```python
from build123d import *

# Parameters (mm, degrees)
F1_DEPTH = 15
F2_DEPTH = 2
F3_R     = 1.8
F4_DEPTH = 50


with BuildPart() as f1:
    # F0 (on Top) → F1 (new body)
    with BuildSketch(Plane.XY):
        Polygon((7.5, -12.990381), (15, 0), (7.5, 12.990381), (-7.5, 12.990381), (-15, 0), (-7.5, -12.990381), align=None)
        Polygon((6.75, 11.691343), (13.5, 0), (6.75, -11.691343), (-6.75, -11.691343), (-13.5, 0), (-6.75, 11.691343), align=None, mode=Mode.SUBTRACT)
    extrude(amount=F1_DEPTH)

    # F0 (on Top) → F2 (join)
    with BuildSketch(Plane.XY):
        Polygon((6.75, -11.691343), (13.5, 0), (6.75, 11.691343), (-6.75, 11.691343), (-13.5, 0), (-6.75, -11.691343), align=None)
    extrude(amount=F2_DEPTH)

    # F3 (on Top) → F4 (join)
    with BuildSketch(Plane.XY):
        with Locations((-11, 0)):
            Circle(F3_R)
        with Locations((5.427412, 9.569215)):
            Circle(F3_R)
        with Locations((5.408632, -9.580663)):
            Circle(F3_R)
        with Locations((0.070379, -0.000349)):
            Circle(F3_R)
    extrude(amount=-F4_DEPTH)


solid = f1.part
```
The listing builds one solid part. Answer for the finished solid, in the listing's coordinates (mm). A direction names the side the tool comes from. Give positions to 0.01 mm unless a question says otherwise; leave off trailing zeros. Order: outer loops, then holes, each group sorted by start corner. A loop starts at its lowest first (then second) coordinate and runs counter-clockwise, first axis right, second up. Notation, with made-up numbers: (-14, 53) -> (30, 53) arc R17 cw to (30, 84) -> close; hole circle Ø2 at (-9, 4). An arc over 180 degrees is marked (long way). One line per item, written item: value.
1) Find section D-D, the plane x = -11. Determine the outline of the cut face in (y, z), plus the area to 3 significant figures.
Reported:
outline: (-6.93, 0) -> (-1.8, 0) -> (-1.8, -50) -> (1.8, -50) -> (1.8, 0) -> (6.93, 0) -> (6.93, 15) -> (4.33, 15) -> (4.33, 2) -> (-4.33, 2) -> (-4.33, 15) -> (-6.93, 15) -> close
area: 275 mm^2
2) Find the intervals of material crossed by line 1 (Y direction, x = -3.5, z = 5); line 2 (X direction, y = -0.25, z = -22); line 3 (Z direction, x = -6, y = 11.5), in increasing order.
Reported:
line 1: y = -12.99 to -11.69, 11.69 to 12.99
line 2: x = -12.78 to -9.22, -1.71 to 1.85
line 3: z = 0 to 2
3) Find section C-C, the plane y = 6.25. Determine the outline of the cut face in (x, z).
Reported:
outline: (-11.39, 0) -> (11.39, 0) -> (11.39, 15) -> (9.89, 15) -> (9.89, 2) -> (-9.89, 2) -> (-9.89, 15) -> (-11.39, 15) -> close
4) Find section B-B, the plane x = -4.5. Determine the outline of the cut face in (y, z).
Reported:
outline: (-12.99, 0) -> (12.99, 0) -> (12.99, 15) -> (11.69, 15) -> (11.69, 2) -> (-11.69, 2) -> (-11.69, 15) -> (-12.99, 15) -> close
5) Find section A-A, the plane z = 7.5. Determine the outline of the cut face in (x, y), plus the area to 3 significant figures.
Reported:
outline: (-15, 0) -> (-7.5, -12.99) -> (7.5, -12.99) -> (15, 0) -> (7.5, 12.99) -> (-7.5, 12.99) -> close; hole (-13.5, 0) -> (-6.75, -11.69) -> (6.75, -11.69) -> (13.5, 0) -> (6.75, 11.69) -> (-6.75, 11.69) -> close
area: 111 mm^2
6) Flat-ended cylindrical pins translate along their axes: P1, Ø1, axis at x = 2, y = 3.5, coming from the -Z side; P2, Ø5, axis at y = 8, z = -33.5, coming from the +X side; P3, Ø5, axis at x = 6.5, z = -3, coming from the +Y side. Find the tip coordinate at first contact, or state that the pin passes through.
Reported:
P1: stops at z = 0
P2: stops at x = 7.23
P3: stops at y = 11.37
7) Determine the mould class of faces 1 (the flat face through (11.302, 6.404, 7.395)), 2 (the flat face through (0, 11.691, 8)), 3 (the cylindrical face through (5.174, -7.796, -24.65)) for opening direction X: pulls with the +X half, pulls with the -X half, needs draft (parallel to the pull), parting line crosses it, or undercut.
Reported:
face 1: pulls with the +X half
face 2: undercut
face 3: parting line crosses it
8) A tool of negligible diameter and unlimited length cuts with its end or side. For faces 4 (the flat face through (-10.078, -5.928, 8.409)), 5 (the cylindrical face through (1.8, 0.5, -24.6)), 6 (the flat face through (11.198, -6.586, 7.395)), from which of +Z, -Z, +X, -X, +Y, -Y can it reach the whole face along a straight path? Write none if from no direction.
Reported:
face 4: +Z
face 5: -Z
face 6: +Z, -Z, +X, -Y
